Geometry: see drawing. Coordinates: mm, zero at the bounding-box minimum. A direction names the side the tool comes from. Coordinates: 2 decimals unless noted, no trailing zeros. Order: outer loops, then holes, each group sorted by start corner. A loop starts at its lowest first (then second) coordinate and runs counter-clockwise, first axis right, second up.
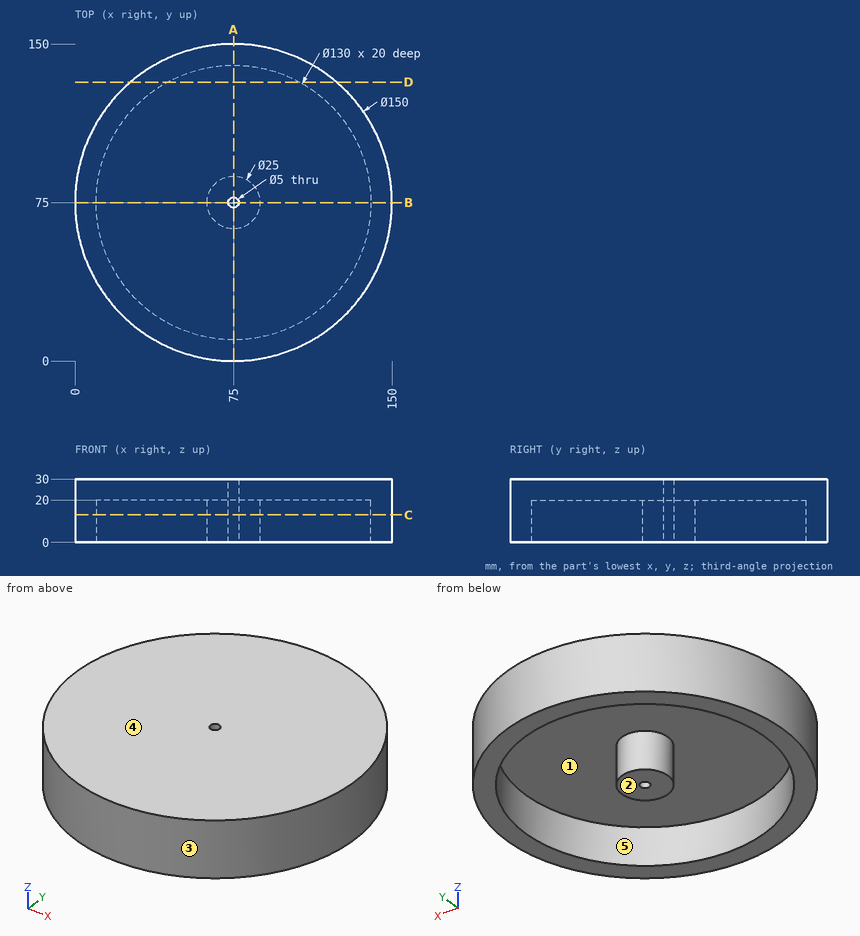
Q1. Pin query (flat end, axial travel): P1, Ø1, axis at y = 123, z = 26.5, coming from the +X side; P2, Ø4, axis at x = 129, z = 15, coming from the +Y side; P3, Ø2, axis at x = 97.5, z = 11, coming from the +Y side; P4, Ø8, axis at x = 75, y = 75, coming from the +Z side. Return the tip coordinate at first contact, or that it passes through.
Solutions:
P1: stops at x = 133.04
P2: stops at y = 129.05
P3: stops at y = 146.85
P4: stops at z = 30
Q2. Section query D-D on y = 132. Output: boundary loops of the cut face in (x, z), plus the area to 3 significant figures.
Solutions:
outline: (26.26, 0) - (43.76, 0) - (43.76, 20) - (106.24, 20) - (106.24, 0) - (123.74, 0) - (123.74, 30) - (26.26, 30) - close
area: 1,680 mm2
Q3. Set-up query: the marked faces 4 and 5. Return all of +Z, -Z, +X, -X, +Y, -Y with unobstructed straight access to the full face (end or side cutting, diameter ignored); none if empty.
Solutions:
face 4: +Z, +X, -X, +Y, -Y
face 5: -Z
Q4. Section query A-A on x = 75. Output: boundary loops of the cut face in (y, z).
Solutions:
outline: (0, 0) - (10, 0) - (10, 20) - (62.5, 20) - (62.5, 0) - (72.5, 0) - (72.5, 30) - (0, 30) - close; (77.5, 0) - (87.5, 0) - (87.5, 20) - (140, 20) - (140, 0) - (150, 0) - (150, 30) - (77.5, 30) - close
Q5. Pull-direction query (X, two-part tool) for the marked faces 1, 2 and 3; classes: pulls with the +X half, pulls with the -X half, needs draft (parallel to the pull), parting line crosses it, or undercut.
Solutions:
face 1: undercut
face 2: needs draft
face 3: parting line crosses it
Q6. Section query C-C on z = 13. Output: boundary loops of the cut face in (x, y), plus the area to 3 significant figures.
Solutions:
outline: circle Ø150 at (75, 75); circle Ø25 at (75, 75); hole circle Ø130 at (75, 75); hole circle Ø5 at (75, 75)
area: 4,870 mm2
Q7. Material intervals for line 1 along Y through (x, z) = (75, 19); line 2 along X through (y, z) = (70.5, 8.75); line 3 along Y through (x, z) = (73.5, 7.5) (3 decimals), sorted ascending.
Solutions:
line 1: y = 0 to 10, 62.5 to 72.5, 77.5 to 87.5, 140 to 150
line 2: x = 0.14 to 10.16, 63.34 to 86.66, 139.84 to 149.86
line 3: y = 0.015 to 10.017, 62.59 to 73, 77 to 87.41, 139.983 to 149.985
